Input: part model. Units: mm. Frame: model coordinates. Coordinates: 2 decimals unless noted, no trailing zeros. Loops run counter-clockwise (first coordinate to the right, second up) from the corner with the lowest first, then second, coordinate; pieces in that order, holes last.
Item 1: Ray query, line 1 along Y through (x, z) = (-3.5, 7.5); line 2 along X through (y, z) = (2, -11.5); line 3 along Y through (x, z) = (-2.25, 117.5). Return the intervals inside material, ascending.
Item 2: Contact query for flat-ended pins moving along their axis: P1, Ø6, axis at x = 1, z = -38.5, coming from the -Y side; P2, Ø1.4, axis at x = -5, z = -3, coming from the +Y side; P3, Ø3, axis at x = -3.5, z = -36, coming from the +Y side. Output: stop coordinate, or through.
Item 3: Section A-A on z = -38. Return loops of the section in (x, y).
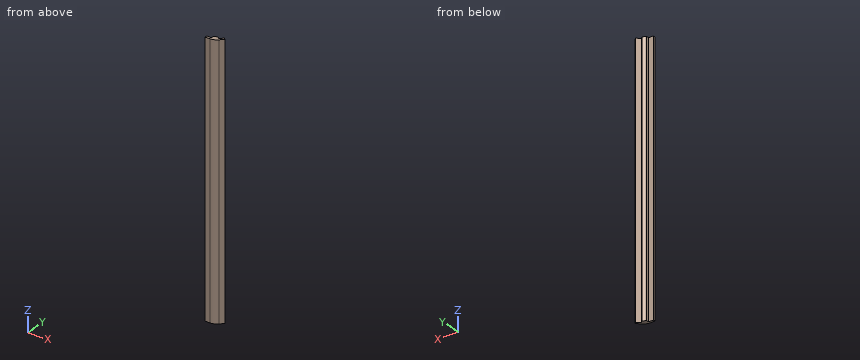
```python
from build123d import *

# Parameters (mm, degrees)
SKETCH7_W           = 4.7625
SKETCH7_H           = 2.12122512
BOSS_EXTRUDE2_DEPTH = 130.175
BOSS_EXTRUDE3_DEPTH = 130.175
BOSS_EXTRUDE4_DEPTH = 130.175


with BuildPart() as part:
    # Sketch7 → Boss-Extrude2 (new, symmetric)
    with BuildSketch(Plane.XY):
        with Locations((-4.92125, -2.560612608)):
            Rectangle(SKETCH7_W, SKETCH7_H)
    extrude(amount=BOSS_EXTRUDE2_DEPTH, both=True)



with BuildPart() as body_2:
    # Sketch8 → Boss-Extrude3 (new, symmetric)
    with BuildSketch(Plane.XY):
        Polygon((2.85671143, 0.735391018), (6.224307475, 4.102987064), (7.724240142, 2.603054397), (4.356644097, -0.764541648), align=None)
    extrude(amount=BOSS_EXTRUDE3_DEPTH, both=True)


with BuildPart() as part_1:
    add(part.part)

    add(body_2.part)  # Boss-Extrude4 merges body 2
    # Sketch11 → Boss-Extrude4 (add, symmetric)
    with BuildSketch(Plane.XY):
        with BuildLine():
            Line((-2.54, -1.500000048), (-7.3025, -1.500000048))
            Line((-7.3025, -1.500000048), (-7.3025, -3.621225168))
            Line((-7.3025, -3.621225168), (-2.54, -3.621225168))
            ThreePointArc((-2.54, -3.621225168), (1.192436889, -2.87879731), (4.356644097, -0.764541648))
            Line((4.356644097, -0.764541648), (7.724240142, 2.603054397))
            Line((7.724240142, 2.603054397), (6.224307475, 4.102987064))
            Line((6.224307475, 4.102987064), (2.85671143, 0.735391018))
            Line((2.85671143, 0.735391018), (0.735391018, 2.85671143))
            ThreePointArc((0.735391018, 2.85671143), (-0.767371154, 1.852597848), (-2.54, 1.500000048))
            Line((-2.54, 1.500000048), (-2.54, -1.500000048))
        make_face()
    extrude(amount=BOSS_EXTRUDE4_DEPTH, both=True)


solid = part_1.part
```
Results found:
1. line 1: y = -3.62 to -1.5
1. line 2: x = -0.45 to 1.59, 4.12 to 7.12
1. line 3: y = -3.62 to 1.51
2. P1: stops at y = -3.61
2. P2: stops at y = -1.5
2. P3: stops at y = 1.53
3. outline: (-7.3, -3.62) - (-2.54, -3.62) arc R9.75 ccw to (4.36, -0.76) - (7.72, 2.6) - (6.22, 4.1) - (2.86, 0.74) - (0.74, 2.86) arc R4.63 cw to (-2.54, 1.5) - (-2.54, -1.5) - (-7.3, -1.5) - close
